Check sheet for the modelled part. Datum: model origin and axes. Units: mm. Face numbers are marked on the shaded views. A direction names the side the tool comes from. Round coordinates to 2 decimals unless told otherwise and drop trailing zeros. Loops run counter-clockwise (first coordinate to the right, second up) from the corner with the lowest first, then second, coordinate; pieces in that order, holes last. Notation, with made-up numbers: (89, 85) - (123, 85) arc R24 cw to (123, 110) - close; hole circle Ø5 at (36, 32). An arc over 180 degrees is marked (long way). Return JSON: item names as keys, results as strings.
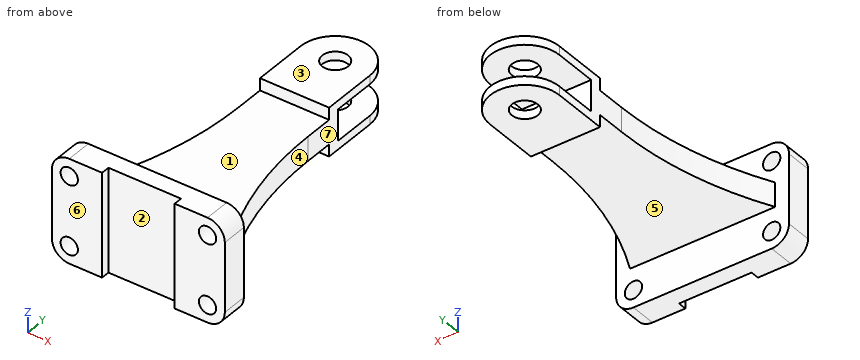
Autodesk Inventor part; units mm, degrees
ref_plane "YZ Plane" through (0, 0, 0) normal (1, 0, 0) x (0, 1, 0)
ref_plane "XZ Plane" through (0, 0, 0) normal (0, 1, 0) x (-1, 0, 0)
ref_plane "XY Plane" through (0, 0, 0) normal (0, 0, 1) x (1, 0, 0)
sketch "Sketch1" plane through (0, 0, 0) normal (0, 1, 0) x (-1, 0, 0)
  line L0 (50, 30) -> (-50, 30)
  line L1 (-50, 30) -> (-50, -30)
  line L2 (-50, -30) -> (50, -30)
  line L3 (50, -30) -> (50, 30)
  line L4 (50, 30) -> (-50, -30) construction
  line L5 (-50, 30) -> (50, -30) construction
  point P0 (0, 0)
  dimension "d0" = 100
  dimension "d1" = 60
extrude "Extrusion1" add sketch "Sketch1" along normal blind 15
fillet "Fillet1" radius 10 4 edges at (50, 7.5, -30) (-50, 7.5, -30) (-50, 7.5, 30) (50, 7.5, 30)
sketch "Sketch2" plane through (0, 0, 0) normal (0, 0, 1) x (1, 0, 0)
  line L0 (40, 0) -> (-40, 0)
  arc A0 (20, 155) -> (-20, 155) centre (0, 155) ccw
  line L1 (-20, 155) -> (-20, 106.1921)
  arc A1 (-42, 15) -> (-20, 106.1921) centre (-220, 106.1921) ccw
  line L2 (40, 15) -> (-40, 15)
  line L3 (0, 155) -> (0, -9.0216)
  line L4 (20, 155) -> (20, 106.1921)
  arc A2 (20, 106.1921) -> (42, 15) centre (220, 106.1921) ccw
  line L5 (-42, 15) -> (42, 15)
  line L6 (-50, 15) -> (-40, 15)
  point P0 (0, 0)
  point P1 (0, 0)
  dimension "d5" = 20
  dimension "d6" = 155
  dimension "d7" = 84
  dimension "d8" = 200
extrude "Extrusion2" add sketch "Sketch2" along normal mid plane 14
sketch "Sketch3" plane through (0, 0, 0) normal (0, 0, 1) x (1, 0, 0)
  line L0 (-20, 106.1921) -> (-20, 155)
  line L1 (-20, 123) -> (20, 123)
  line L2 (20, 155) -> (20, 106.1921)
  arc A0 (20, 155) -> (-20, 155) centre (0, 155) ccw
  line L3 (-20, 155) -> (-20, 123)
  line L4 (20, 123) -> (20, 155)
  point P0 (0, 0)
  dimension "d11" = 32
extrude "Extrusion3" add sketch "Sketch3" along normal mid plane 28
sketch "Sketch4" plane through (20, 106.1921, 7) normal (1, 0, 0) x (0, 0, -1)
  line L0 (0, 0) -> (14, 0)
  line L1 (21, 48.8079) -> (-7, 48.8079)
  line L2 (-2, 68.8079) -> (16, 68.8079)
  line L3 (16, 68.8079) -> (16, 23.8079)
  line L4 (16, 23.8079) -> (-2, 23.8079)
  line L5 (-2, 23.8079) -> (-2, 68.8079)
  line L6 (21, 68.8079) -> (-7, 68.8079)
  point P0 (7, -106.1921)
  point P1 (7, 23.8079)
  point P2 (7, 0)
  dimension "d14" = 25
  dimension "d15" = 18
extrude "Extrusion4" cut sketch "Sketch4" against normal through all
sketch "Sketch5" plane through (-40, 0, 30) normal (0, 0, 1) x (1, 0, 0)
  line L0 (0, 0) -> (80, 0)
  line L1 (19, 5) -> (61, 5)
  line L2 (61, 5) -> (61, 0)
  line L3 (61, 0) -> (19, 0)
  line L4 (19, 0) -> (19, 5)
  point P0 (40, 0)
  point P1 (40, 0)
  point P2 (61, 0)
  dimension "d18" = 42
  dimension "d19" = 5
extrude "Extrusion5" cut sketch "Sketch5" against normal through all
sketch "Sketch6" plane through (0, 0, 14) normal (0, 0, 1) x (1, 0, 0)
  arc A0 (20, 155) -> (-20, 155) centre (0, 155) ccw
  point P0 (0, 0)
hole "Hole1" at (0, 155, 14) direction (0, 0, -1) diameter 15 end through all
sketch "Sketch7" plane through (0, 15, 0) normal (0, 1, 0) x (1, 0, 0)
  arc A0 (40, -30) -> (50, -20) centre (40, -20) ccw
  arc A1 (50, 20) -> (40, 30) centre (40, 20) ccw
  arc A2 (-40, 30) -> (-50, 20) centre (-40, 20) ccw
  arc A3 (-50, -20) -> (-40, -30) centre (-40, -20) ccw
  point P0 (0, 0)
hole "Hole2" at (-40, 15, -20) at (-40, 15, 20) at (40, 15, -20) at (40, 15, 20) direction (0, -1, 0) diameter 10 end through all
properties part number "Part012. HighStand" material "Steel, Cast"
Q1. Sectioned sample at C-C (z = -5). Enter the section's corners in (x, y).
Answer key:
{"outline": "(-50, 0) - (-21, 0) - (-21, 5) - (21, 5) - (21, 0) - (50, 0) - (50, 15) - (42, 15) arc R200 cw to (20, 106.19) - (20, 130) - (-20, 130) - (-20, 106.19) arc R200 cw to (-42, 15) - (-50, 15) - close"}
Q2. Sectioned sample at D-D (x = -16). Enter the section's corners in (y, z), plus the area to 3 significant figures.
Answer key:
{"outline": "(5, -30) - (15, -30) - (15, -7) - (123, -7) - (123, -14) - (167, -14) - (167, -9) - (130, -9) - (130, 9) - (167, 9) - (167, 14) - (123, 14) - (123, 7) - (15, 7) - (15, 30) - (5, 30) - close", "area": "2,680 mm²"}
Q3. Sectioned sample at A-A (z = 11). Enter the section's corners in (x, y), plus the area to 3 significant figures.
Answer key:
{"outline": "(-50, 0) - (-21, 0) - (-21, 5) - (21, 5) - (21, 0) - (50, 0) - (50, 15) - (-50, 15) - close; (-20, 123) - (20, 123) - (20, 155) arc R20 ccw to (-20, 155) - close; hole circle Ø15 at (0, 155)", "area": "3,020 mm²"}
Q4. Sectioned sample at B-B (x = 0). Enter the section's corners in (y, z).
Answer key:
{"outline": "(5, -30) - (15, -30) - (15, -7) - (123, -7) - (123, -14) - (147.5, -14) - (147.5, -9) - (130, -9) - (130, 9) - (147.5, 9) - (147.5, 14) - (123, 14) - (123, 7) - (15, 7) - (15, 30) - (5, 30) - close; (162.5, -14) - (175, -14) - (175, -9) - (162.5, -9) - close; (162.5, 9) - (175, 9) - (175, 14) - (162.5, 14) - close"}
Q5. Scan lines: probe 1 along Y at (x, z) = (0, -12); probe 2 along X at (y, z) = (9, -20); probe 3 along Z at (x, y) = (-40, 6). Record each from-to range of solid material in increasing order. Write a range as [from, to].
Answer key:
{"probe 1": "y = [5, 15], [123, 147.5], [162.5, 175]", "probe 2": "x = [-50, -45], [-35, 35], [45, 50]", "probe 3": "z = [-30, -25], [-15, 15], [25, 30]"}
Q6. Draft check along Y on the marked faces 4, 5, 6 and 7. Enter one of: released by +Y, released by -Y, zero draft, split by the parting line, or undercut.
Answer key:
{"face 4": "released by +Y", "face 5": "undercut", "face 6": "released by -Y", "face 7": "zero draft"}
Q7. Depth check by flat-ended pin: P1, Ø10, axis at y = 89.5, z = 4, coming from the +X side; P2, Ø12, axis at x = -8, y = 155, coming from the +Z side; P3, Ø2, axis at x = 10, z = -9.5, coming from the -Y side. Enter the tip coordinate at first touch or a pass-through.
Answer key:
{"P1": "stops at x = 21.18", "P2": "stops at z = 14", "P3": "stops at y = 5"}
Q8. Tool access check on the marked faces 1, 2 and 3. Record the directions out of +Z, -Z, +X, -X, +Y, -Y that give a thin tool (end or side, any length) a straight path to the whole face; none if there is none.
Answer key:
{"face 1": "+Z, +X, -X", "face 2": "+Z, -Z, -Y", "face 3": "+Z, +X, -X, +Y"}
